```python
from build123d import *

# Parameters (mm, degrees)
F0_W     = 280
F0_H     = 110
F1_DEPTH = 160
F2_T     = -10
F3_W     = 260
F3_H     = 90
F3_W_2   = 108
F3_H_2   = 16
F3_W_3   = 14
F4_DEPTH = 150
F5_DEPTH = 40
F6_R     = 9
F7_DEPTH = 25


with BuildPart() as f1:
    # F0 (on Top) → F1 (new body)
    with BuildSketch(Plane.XY):
        Rectangle(F0_W, F0_H)
    extrude(amount=F1_DEPTH)

    # F2
    f2_openings = [f1.faces().sort_by_distance(p)[0] for p in [
        (0, 0, 160),
    ]]
    offset(amount=F2_T, openings=f2_openings)

    # F3 (on face) → F4 (join)
    with BuildSketch(Plane.XY.offset(10)):
        Rectangle(F3_W, F3_H)
        Polygon((115, 30), (115, 24.33777228), (115, 8), (115, -8), (115, -26.8225744367), (115, -30), (7, -30), (-7, -30), (-115, -30), (-115, -8), (-115, 8), (-115, 30), (-15, 30), (-7, 30), (7, 30), align=None, mode=Mode.SUBTRACT)
        with Locations((61, 0)):
            Rectangle(F3_W_2, F3_H_2)
        Polygon((-7, -8), (-7, 8), (-109.6588596702, 8), (-115, 8), (-115, -8), (-109.6588596702, -8), align=None)
        Polygon((-7, 8), (7, 8), (7, 30), (-7, 30), (-7, 15.2422059327), align=None)
        Polygon((7, -16.3514893502), (7, -8), (-7, -8), (-7, -30), (7, -30), align=None)
        Rectangle(F3_W_3, F3_H_2)
    extrude(amount=F4_DEPTH)

    # F3 (on face) → F5 (join)
    with BuildSketch(Plane.XY.offset(10)):
        Rectangle(F3_W, F3_H)
        Polygon((115, 30), (115, 24.33777228), (115, 8), (115, -8), (115, -26.8225744367), (115, -30), (7, -30), (-7, -30), (-115, -30), (-115, -8), (-115, 8), (-115, 30), (-15, 30), (-7, 30), (7, 30), align=None, mode=Mode.SUBTRACT)
        Polygon((115, 8), (115, 24.33777228), (115, 30), (7, 30), (7, 8), align=None)
        Polygon((115, -26.8225744367), (115, -8), (7, -8), (7, -16.3514893502), (7, -30), (115, -30), align=None)
        Polygon((-109.6588596702, 8), (-7, 8), (-7, 15.2422059327), (-7, 30), (-15, 30), (-115, 30), (-115, 8), align=None)
        Polygon((-7, -30), (-7, -8), (-109.6588596702, -8), (-115, -8), (-115, -30), align=None)
        with Locations((61, 0)):
            Rectangle(F3_W_2, F3_H_2)
        Polygon((-7, -8), (-7, 8), (-109.6588596702, 8), (-115, 8), (-115, -8), (-109.6588596702, -8), align=None)
        Rectangle(F3_W_3, F3_H_2)
    extrude(amount=F5_DEPTH)

    # F6 (on face) → F7 (cut)
    with BuildSketch(Plane(origin=(-140, 0, 0), x_dir=(0, -1, 0), z_dir=(-1, 0, 0))):
        with Locations((0, 25.6529357284)):
            Circle(F6_R)
    extrude(amount=-F7_DEPTH, mode=Mode.SUBTRACT)


solid = f1.part
```
Check sheet for the modelled part. Datum: model origin and axes. Units: mm. A direction names the side the tool comes from. Round coordinates to 2 decimals unless told otherwise and drop trailing zeros. Loops run counter-clockwise (first coordinate to the right, second up) from the corner with the lowest first, then second, coordinate; pieces in that order, holes last. Notation, with made-up numbers: (87, -27) -> (98, -27) arc R32 ccw to (98, 3) -> close; hole circle Ø9 at (64, -9.75). An arc over 180 degrees is marked (long way). Write item = value, one per line. Start each with the question number.
1) Gauge pin test, flat end, axial feed: pin 1 Ø11 at (y, z) = (0, 25.65) entering from -X. Record the tip position at first contact, or that the pin passes through.
2) Sectioned sample at A-A, the plane z = 72. Record the cut outline in (x, y).
3) Sectioned sample at B-B, the plane y = 13.5. Record the cut outline in (x, z).
4) Release check for a two-part mould opening along X. For faces 4 (the flat face through (-62, -19, 50)), 5 (the flat face through (140, -1, 79)), 6 (the flat face through (-2, 55, 79)) record: released by +X, released by -X, zero draft, split by the parting line, or undercut.
5) Thickness scan on probe 1 along Y at (x, z) = (-57, 140); probe 2 along X at (y, z) = (-22, 58.5); probe 3 along Z at (x, y) = (-122, 0). Record the ranges inside material, lowest first.
6) Sectioned sample at C-C, the plane x = 50.5. Record the cut outline in (y, z).
7) Set-up check for faces 1 (the flat face through (-2, 1, 0)), 2 (the cylindrical face through (-127.675, 1.172, 34.576)), 3 (the flat face through (-60, 8, 104)): record each of +Z, -Z, +X, -X, +Y, -Y from which the full face is reachable in a straight line by a thin tool's end or side.
Results are:
q1.pin_1 = -115
q2.outline = (-140, -55) -> (140, -55) -> (140, 55) -> (-140, 55) -> close; hole (-115, -30) -> (-7, -30) -> (-7, -8) -> (-115, -8) -> close; hole (-115, 8) -> (-7, 8) -> (-7, 30) -> (-115, 30) -> close; hole (7, -30) -> (115, -30) -> (115, -8) -> (7, -8) -> close; hole (7, 8) -> (115, 8) -> (115, 30) -> (7, 30) -> close
q3.outline = (-140, 0) -> (140, 0) -> (140, 160) -> (115, 160) -> (115, 50) -> (7, 50) -> (7, 160) -> (-7, 160) -> (-7, 50) -> (-115, 50) -> (-115, 160) -> (-140, 160) -> close
q4.face_4 = undercut
q4.face_5 = released by +X
q4.face_6 = zero draft
q5.probe_1 = -55 to -30, -8 to 8, 30 to 55
q5.probe_2 = -140 to -115, -7 to 7, 115 to 140
q5.probe_3 = 0 to 16.65, 34.65 to 160
q6.outline = (-55, 0) -> (55, 0) -> (55, 160) -> (30, 160) -> (30, 50) -> (8, 50) -> (8, 160) -> (-8, 160) -> (-8, 50) -> (-30, 50) -> (-30, 160) -> (-55, 160) -> close
q7.face_1 = -Z, +X, -X, +Y, -Y
q7.face_2 = -X
q7.face_3 = +Z
